Read the model definition and answer for the solid it produces. Units are mm, in the model's axes. Face numbers are marked on the shaded views. A direction names the side the tool comes from. Coordinates: 2 decimals unless noted, no trailing zeros. Write each loop counter-clockwise with the first axis right and the second up, starting at its lowest first coordinate (ties: lowest second). Pieces come first, ordered by that corner, then holes. Notation, with made-up numbers: M 15,-32.5 L 62,-32.5 A16 ccw 62,-25.5 Z; hole C 25.25,-36 d6. An arc over 180 degrees is marked long. Write item = value, one per line.
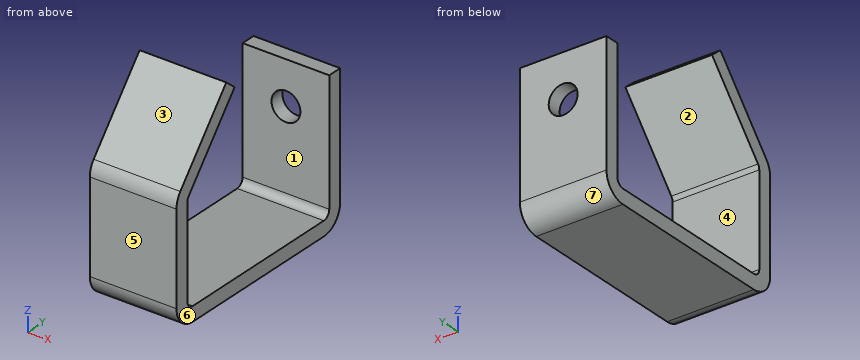
from build123d import *

# Parameters (mm, degrees)
BOSS_EXTRUDE1_DEPTH = 19.05
SHELL1_T            = 6.35
FILLET1_R           = 3.175
FILLET2_R           = 9.525
CUT_EXTRUDE1_REACH  = 128.663
SKETCH2_R           = 6.35


with BuildPart() as part:
    # Sketch1 → Boss-Extrude1 (new, symmetric)
    with BuildSketch(Plane(origin=(0, 0, 0), x_dir=(0, 0, -1), z_dir=(1, 0, 0))):
        Polygon((-57.15, 82.55), (0, 82.55), (0, 0), (-44.45, 0), (-77.208974413, 27.488043348), (-57.15, 51.393398168), align=None)
    extrude(amount=BOSS_EXTRUDE1_DEPTH, both=True)

    # Shell1
    shell1_openings = [part.faces().sort_by_distance(p)[0] for p in [
        (19.05, 40.856533518, 31.097326269),
        (0, 39.440720758, 67.179487206),
        (-19.05, 40.856533518, 31.097326269),
        (0, 66.971699084, 57.15),
    ]]
    offset(amount=SHELL1_T, openings=shell1_openings, kind=Kind.INTERSECTION)

    # Fillet1
    # the kernel refuses this fillet: 3.175 mm, written as the material it adds along each edge
    with BuildSketch(Plane(origin=(19.05, 0, 0), x_dir=(0, 0, 1), z_dir=(-1, 0, 0)), Plane(origin=(19.05, 82.55, 0), x_dir=(0, -1, 0), z_dir=(-1, 0, 0))) as fillet1_piece_1:
        with BuildLine():
            CenterArc((FILLET1_R, FILLET1_R), FILLET1_R, 180, 90)
            Line((0, FILLET1_R), (0, 0))
            Line((0, 0), (FILLET1_R, 0))
        make_face()
    extrude(amount=38.1)
    with BuildSketch(Plane(origin=(19.05, 0, 44.45), x_dir=(0, 0.6427876096865391, 0.7660444431189782), z_dir=(-1, 0, 0))) as fillet1_piece_2:
        with BuildLine():
            CenterArc((FILLET1_R * 0.363970234266, FILLET1_R), FILLET1_R, 230, 40)
            Line((-FILLET1_R * 0.27881737542, FILLET1_R * 0.233955556881), (0, 0))
            Line((0, 0), (FILLET1_R * 0.363970234266, 0))
        make_face()
    extrude(amount=38.1)

    # Fillet2
    fillet2_edges = [part.edges().sort_by_distance(p)[0] for p in [
        (0, -6.35, 46.761210988),
        (0, -6.35, -6.35),
        (0, 88.9, -6.35),
    ]]
    fillet(fillet2_edges, radius=FILLET2_R)

    # Sketch2 → Cut-Extrude1 (cut, up to next)
    with BuildSketch(Plane(origin=(0, 88.9, 0), x_dir=(-1, 0, 0), z_dir=(0, 1, 0)), mode=Mode.PRIVATE) as cut_extrude1_sk1:
        with Locations(Location((0, 38.1, 0), (0, 0, 90))):
            Circle(SKETCH2_R)
    cut_extrude1_tool1 = extrude(cut_extrude1_sk1.sketch, amount=-CUT_EXTRUDE1_REACH, mode=Mode.PRIVATE) & part.part
    add(cut_extrude1_tool1.solids().sort_by_distance((0, 88.9, 38.1))[0], mode=Mode.SUBTRACT)


solid = part.part
Item 1: Find section D-D (y = 4.5). Determine the outline of the cut face in (x, z).
Worked answers:
outline = M -19.05,-6.35 L 19.05,-6.35 L 19.05,0 L -19.05,0 Z; M -19.05,49.81 L 19.05,49.81 L 19.05,59.69 L -19.05,59.69 Z
Item 2: Find section C-C (z = 21.5). Determine the outline of the cut face in (x, y), and give its area (3 significant figures).
Worked answers:
outline = M -19.05,-6.35 L 19.05,-6.35 L 19.05,0 L -19.05,0 Z; M -19.05,82.55 L 19.05,82.55 L 19.05,88.9 L -19.05,88.9 Z
area = 484 mm²
Item 3: Find section B-B (x = 0). Determine the outline of the cut face in (y, z) (3 decimals), and give its area (3 significant figures).
Worked answers:
outline = M -6.35,3.175 A9.525 ccw 3.175,-6.35 L 79.375,-6.35 A9.525 ccw 88.9,3.175 L 88.9,31.75 L 82.55,31.75 L 82.55,3.175 A3.175 cw 79.375,0 L 3.175,0 A3.175 cw 0,3.175 L 0,43.294 A3.175 cw 0.743,45.335 L 27.488,77.209 L 22.624,81.291 L -4.122,49.417 A9.525 ccw -6.35,43.294 Z; M 82.55,44.45 L 88.9,44.45 L 88.9,57.15 L 82.55,57.15 Z
area = 1,420 mm²
Item 4: Find section A-A (z = 38.1). Determine the outline of the cut face in (x, y).
Worked answers:
outline = M -19.05,-6.35 L 19.05,-6.35 L 19.05,0 L -19.05,0 Z; M -19.05,82.55 L -6.35,82.55 L -6.35,88.9 L -19.05,88.9 Z; M 6.35,82.55 L 19.05,82.55 L 19.05,88.9 L 6.35,88.9 Z
Item 5: Flat-ended cylindrical pins translate along their axes: pin 1 (12 mm diameter, centred on x = -14.5, z = 54, fed in from -Y); pin 2 (8 mm diameter, centred on x = -2, z = 64, fed in from -Y); pin 3 (11.5 mm diameter, centred on x = -3, y = 39, fed in from +Z). Find the tip coordinate at first contact, or state that the pin passes through.
Worked answers:
pin_1 = -5.11
pin_2 = 4.76
pin_3 = 0
Item 6: For a pull along Y with two mould halves and no side action, classify the marked faces 4, 5, 6 and 7 as released by +Y, released by -Y, zero draft, split by the parting line, or undercut.
Worked answers:
face_4 = undercut
face_5 = released by -Y
face_6 = zero draft
face_7 = released by +Y
Item 7: Consider line 1 along X through (y, z) = (84, 38); line 2 along Y through (x, z) = (-12, 5). Determine where each line is inside the solid, lowest interval first. Write a range as from..to.
Worked answers:
line_1 = -19.05..-6.35, 6.35..19.05
line_2 = -6.35..0, 82.55..88.9
Item 8: Which of the six approach directions +Z, -Z, +X, -X, +Y, -Y give full straight-line access (tool end or side, diameter ignored) to the marked faces 1, 2 and 3?
Worked answers:
face_1 = +Z, +X, -X
face_2 = +X, -X
face_3 = +Z, +X, -X, -Y
